Verification items for the finished model (mm, model axes). A direction names the side the tool comes from. Coordinates: 2 decimals unless noted, no trailing zeros. Order: outer loops, then holes, each group sorted by start corner. A loop starts at its lowest first (then second) coordinate and runs counter-clockwise, first axis right, second up. Notation, with made-up numbers: M -14.5,31.25 L -9.5,31.25 A22 ccw -9.5,39.25 Z; hole C 77,-36 d8. An arc over 180 degrees is marked long. Write item = value, one per line.
```python
from build123d import *

# Parameters (mm, degrees)
F0_W     = 1.5
F0_H     = 1.5
F0_H_2   = 23.5
F0_W_2   = 23.5
F1_DEPTH = 100
F3_DEPTH = 1.5


with BuildPart() as f1:
    # F0 (on Top) → F1 (new body)
    with BuildSketch(Plane.XY):
        with Locations((11.75, 0)):
            Rectangle(F0_W, F0_H)
        with Locations((11.75, 12.5)):
            Rectangle(F0_W, F0_H_2)
        with Locations((-0.75, 0)):
            Rectangle(F0_W_2, F0_H)
    extrude(amount=-F1_DEPTH)

    # F2 (on face) → F3 (cut)
    with BuildSketch(Plane.XZ.offset(0.75)):
        with BuildLine():
            Line((-12.5, -56), (-4.5, -56))
            ThreePointArc((-4.5, -56), (1.5, -50), (-4.5, -44))
            Line((-4.5, -44), (-12.5, -44))
            Line((-12.5, -44), (-12.5, -56))
        make_face()
    extrude(amount=-F3_DEPTH, mode=Mode.SUBTRACT)


solid = f1.part
```
Item 1: Sectioned sample at D-D, the plane z = -50. Enter the section's corners in (x, y), then the cut area to 4 significant figures.
Report:
outline = M 1.5,-0.75 L 12.5,-0.75 L 12.5,24.25 L 11,24.25 L 11,0.75 L 1.5,0.75 Z
area = 51.75 mm^2
Item 2: Sectioned sample at B-B, the plane y = 17.5. Enter the section's corners in (x, z).
Report:
outline = M 11,-100 L 12.5,-100 L 12.5,0 L 11,0 Z
Item 3: Scan lines: L1, parallel to X at y = 4, z = -15; L2, parallel to Y at x = -7.5, z = -86. Record each from-to range of solid material in increasing order. Write a range as from..to.
Report:
L1 = 11..12.5
L2 = -0.75..0.75
Item 4: Sectioned sample at C-C, the plane x = 4. Enter the section's corners in (y, z), then the cut area to 3 significant figures.
Report:
outline = M -0.75,-100 L 0.75,-100 L 0.75,0 L -0.75,0 Z
area = 150 mm^2
Item 5: Tool access check on faces 1 (the flat face through (2, 0.75, -49)), 2 (the flat face through (12.5, 12, -49)). Record the directions out of +Z, -Z, +X, -X, +Y, -Y that give a thin tool (end or side, any length) a straight path to the whole face; none if there is none.
Report:
face_1 = +Z, -Z, -X, +Y
face_2 = +Z, -Z, +X, +Y, -Y
Item 6: Release check for a two-part mould opening along Z. For faces 3 (the flat face through (11, 13, -49)), 4 (the cylindrical face through (1.5, 0, -50.1)) record: pulls with the +Z half, pulls with the -Z half, needs draft (parallel to the pull), parting line crosses it, or undercut.
Report:
face_3 = needs draft
face_4 = undercut
Item 7: Sectioned sample at A-A, the plane z = -37. Enter the section's corners in (x, y).
Report:
outline = M -12.5,-0.75 L 12.5,-0.75 L 12.5,24.25 L 11,24.25 L 11,0.75 L -12.5,0.75 Z
Item 8: Gauge pin test, flat end, axial feed: pin 1 (8 mm diameter, centred on y = 17, z = -40, fed in from -X). Record the tip position at first contact, or that the pin passes through.
Report:
pin_1 = 11
